Model file for the job. Use its own axes, mm. Round coordinates to 2 decimals unless told otherwise and drop trailing zeros. Order: outer loops, then holes, each group sorted by start corner. A loop starts at its lowest first (then second) coordinate and runs counter-clockwise, first axis right, second up. Notation, with made-up numbers: (85.25, 0.5) - (117.25, 0.5) arc R26 ccw to (117.25, 35.5) - close; hole circle Ø8 at (8, 30.5). An arc over 180 degrees is marked (long way). Write item = value, one per line.
```python
from build123d import *

# Parameters (mm, degrees)
ESQUISSE1_W        = 105
ESQUISSE1_H        = 46
ESQUISSE1_R        = 2
ESQUISSE1_W_2      = 4
ESQUISSE1_H_2      = 7
BOSS_EXTRU_1_DEPTH = 5
CONG_1_R           = 10


with BuildPart() as part:
    # Esquisse1 → Boss.-Extru.1 (new body)
    with BuildSketch(Plane.XY):
        with Locations((52.5, 23)):
            Rectangle(ESQUISSE1_W, ESQUISSE1_H)
        with Locations((15, 6)):
            Circle(ESQUISSE1_R, mode=Mode.SUBTRACT)
        with Locations((15, 40)):
            Circle(ESQUISSE1_R, mode=Mode.SUBTRACT)
        with Locations((40, 40)):
            Circle(ESQUISSE1_R, mode=Mode.SUBTRACT)
        with Locations((40, 6)):
            Circle(ESQUISSE1_R, mode=Mode.SUBTRACT)
        with Locations((65, 40)):
            Circle(ESQUISSE1_R, mode=Mode.SUBTRACT)
        with Locations((65, 6)):
            Circle(ESQUISSE1_R, mode=Mode.SUBTRACT)
        with Locations((90, 40)):
            Circle(ESQUISSE1_R, mode=Mode.SUBTRACT)
        with Locations((90, 6)):
            Circle(ESQUISSE1_R, mode=Mode.SUBTRACT)
        with Locations((40, 16.5)):
            Rectangle(ESQUISSE1_W_2, ESQUISSE1_H_2, mode=Mode.SUBTRACT)
        with Locations((15, 16.5)):
            Rectangle(ESQUISSE1_W_2, ESQUISSE1_H_2, mode=Mode.SUBTRACT)
        with Locations((65, 16.5)):
            Rectangle(ESQUISSE1_W_2, ESQUISSE1_H_2, mode=Mode.SUBTRACT)
        with Locations((90, 16.5)):
            Rectangle(ESQUISSE1_W_2, ESQUISSE1_H_2, mode=Mode.SUBTRACT)
    extrude(amount=BOSS_EXTRU_1_DEPTH)

    # Congé1
    cong_1_edges = [part.edges().sort_by_distance(p)[0] for p in [
        (0, 46, 2.5),
        (105, 46, 2.5),
        (105, 0, 2.5),
        (0, 0, 2.5),
    ]]
    fillet(cong_1_edges, radius=CONG_1_R)


solid = part.part
```
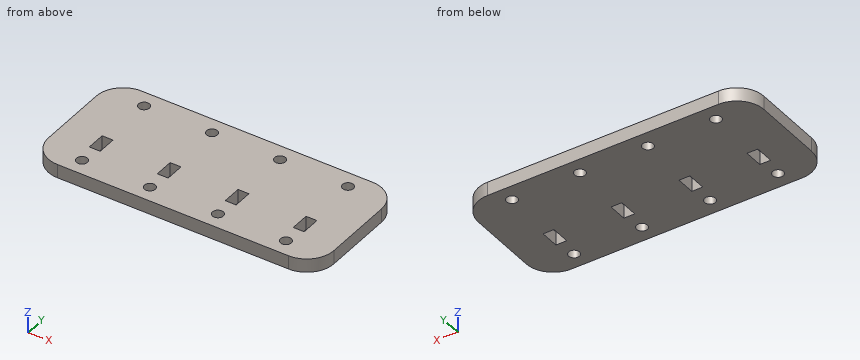
1) Cut at B-B (y = 15.5). Write the cut outline in (x, z), and give its area (3 significant figures).
Conclusion:
outline = (0, 0) - (13, 0) - (13, 5) - (0, 5) - close; (17, 0) - (38, 0) - (38, 5) - (17, 5) - close; (42, 0) - (63, 0) - (63, 5) - (42, 5) - close; (67, 0) - (88, 0) - (88, 5) - (67, 5) - close; (92, 0) - (105, 0) - (105, 5) - (92, 5) - close
area = 445 mm^2
2) Flat gauge pins, fed straight in: pin 1 Ø3 at (x, y) = (65, 6) entering from +Z; pin 2 Ø2 at (y, z) = (8.5, 4) entering from -X. Where does each tip first touch, or does it go through?
Conclusion:
pin_1 = through
pin_2 = 0.01
3) Cut at D-D (y = 5). Write the cut outline in (x, z).
Conclusion:
outline = (1.34, 0) - (13.27, 0) - (13.27, 5) - (1.34, 5) - close; (16.73, 0) - (38.27, 0) - (38.27, 5) - (16.73, 5) - close; (41.73, 0) - (63.27, 0) - (63.27, 5) - (41.73, 5) - close; (66.73, 0) - (88.27, 0) - (88.27, 5) - (66.73, 5) - close; (91.73, 0) - (103.66, 0) - (103.66, 5) - (91.73, 5) - close
4) Cut at C-C (z = 4.1). Give the number of separate pieces and of enclosed holes in the cut face, and give its area (3 significant figures).
Conclusion:
separate_pieces = 1
enclosed_holes = 12
area = 4,530 mm^2
5) Cut at A-A (x = 90). Write the cut outline in (y, z), and give its area (3 significant figures).
Conclusion:
outline = (0, 0) - (4, 0) - (4, 5) - (0, 5) - close; (8, 0) - (13, 0) - (13, 5) - (8, 5) - close; (20, 0) - (38, 0) - (38, 5) - (20, 5) - close; (42, 0) - (46, 0) - (46, 5) - (42, 5) - close
area = 155 mm^2
6) Wall check: line 1 along Y through (x, z) = (15, 1.5); line 2 along X through (y, z) = (39, 0.2); line 3 along X through (y, z) = (4.5, 0.75). Give the ranges that are in metal, low to high.
Conclusion:
line_1 = 0 to 4, 8 to 13, 20 to 38, 42 to 46
line_2 = 0.46 to 13.27, 16.73 to 38.27, 41.73 to 63.27, 66.73 to 88.27, 91.73 to 104.54
line_3 = 1.65 to 13.68, 16.32 to 38.68, 41.32 to 63.68, 66.32 to 88.68, 91.32 to 103.35
